Work out the finished part from the listing and answer in its coordinate system (mm). Face numbers are marked on the shaded views. A direction names the side the tool comes from. Give positions to 0.01 mm unless a question says otherwise; leave off trailing zeros. Loops run counter-clockwise (first coordinate to the right, second up) from the corner with the lowest first, then second, coordinate; pieces in that order, holes last. Notation, with made-up numbers: (65, -35.5) - (88, -35.5) arc R15 cw to (88, -13.5) - close; hole circle Ø6 at (47, -9.75). An arc over 180 degrees is marked (long way). One line per item, written item: value.
from build123d import *

# Parameters (mm, degrees)
SKETCH1_W               = 48
SKETCH1_H               = 40
BOSS_EXTRUDE1_DEPTH     = 6
CUT_EXTRUDE1_DEPTH      = 34.466401061
CUT_EXTRUDE1_DEPTH_BACK = 34.466401061
SKETCH3_R               = 1.5
BOSS_EXTRUDE2_DEPTH     = 1.5
FILLET1_R               = 3


with BuildPart() as part:
    # Sketch1 → Boss-Extrude1 (new, symmetric)
    with BuildSketch(Plane(origin=(0, 0, 0), x_dir=(1, 0, 0), z_dir=(0, 1, 0))):
        Rectangle(SKETCH1_W, SKETCH1_H)
    extrude(amount=BOSS_EXTRUDE1_DEPTH, both=True)

    # Sketch2 → Cut-Extrude1 (cut, two sides: drawn at the far end of the back side and taken through both)
    with BuildSketch(Plane(origin=(0, 6, 0), x_dir=(1, 0, 0), z_dir=(0, 1, 0)).offset(-CUT_EXTRUDE1_DEPTH_BACK)):
        with BuildLine():
            Line((-24, 13), (-20.5, 13))
            ThreePointArc((-20.5, 13), (-18.025126266, 14.025126266), (-17, 16.5))
            Line((-17, 16.5), (-17, 20))
            Line((-17, 20), (-24, 20))
            Line((-24, 20), (-24, 13))
        make_face()
        with BuildLine():
            Line((24, -13), (20.5, -13))
            ThreePointArc((20.5, -13), (18.025126266, -14.025126266), (17, -16.5))
            Line((17, -16.5), (17, -20))
            Line((17, -20), (24, -20))
            Line((24, -20), (24, -13))
        make_face()
    extrude(amount=CUT_EXTRUDE1_DEPTH + CUT_EXTRUDE1_DEPTH_BACK, mode=Mode.SUBTRACT)

    # Sketch3 → Boss-Extrude2 (add, symmetric)
    # profile 1 of 2: a face of its own
    with BuildSketch(Plane(origin=(0, 0, 0), x_dir=(1, 0, 0), z_dir=(0, 1, 0))):
        with BuildLine():
            Line((24, -13), (20.5, -13))
            ThreePointArc((20.5, -13), (18.025126266, -14.025126266), (17, -16.5))
            Line((17, -16.5), (17, -20))
            Line((17, -20), (24, -20))
            Line((24, -20), (24, -13))
        make_face()
        with Locations(Location((20.5, -16.5, 0), (0, 0, 270))):
            Circle(SKETCH3_R, mode=Mode.SUBTRACT)
    # profile 2 of 2: a face of its own
    with BuildSketch(Plane(origin=(0, 0, 0), x_dir=(1, 0, 0), z_dir=(0, 1, 0))):
        with BuildLine():
            Line((-24, 13), (-20.5, 13))
            ThreePointArc((-20.5, 13), (-18.025126266, 14.025126266), (-17, 16.5))
            Line((-17, 16.5), (-17, 20))
            Line((-17, 20), (-24, 20))
            Line((-24, 20), (-24, 13))
        make_face()
        with Locations(Location((-20.5, 16.5, 0), (0, 0, 270))):
            Circle(SKETCH3_R, mode=Mode.SUBTRACT)
    extrude(amount=BOSS_EXTRUDE2_DEPTH, both=True)

    # Fillet1
    fillet1_edges = [part.edges().sort_by_distance(p)[0] for p in [
        (24, 0, 20),
        (-24, 0, 20),
        (24, 0, -20),
        (-24, 0, -20),
    ]]
    fillet(fillet1_edges, radius=FILLET1_R)


solid = part.part
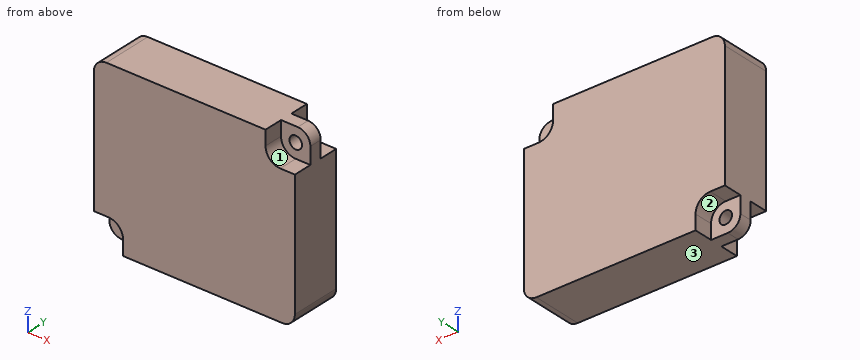
1. For the marked faces 1, 2 and 3, determine the directions among +Z, -Z, +X, -X, +Y, -Y from which every point of the face is accessible in a straight line to the end or side of a thin tool.
Output:
face 1: +Z, +X, -Y
face 2: -Z, -X, +Y
face 3: -Z, +X, -X, +Y, -Y
2. Flat-ended cylindrical pins translate along their axes: pin 1 Ø2.5 at (x, z) = (20.5, 16.5) entering from -Y; pin 2 Ø1 at (y, z) = (-3, -18.5) entering from -X; pin 3 Ø2 at (x, z) = (20.5, 18) entering from -Y; pin 4 Ø1 at (x, y) = (-22.5, -3) entering from -Z. Find the tip coordinate at first contact, or state that the pin passes through.
Output:
pin 1: passes through
pin 2: stops at x = -17
pin 3: stops at y = -1.5
pin 4: stops at z = -13
3. Section B-B (x = -18) is taken. Write down the section's boundary in (y, z), and give its area (3 significant figures).
Output:
outline: (-6, -14.05) - (-1.5, -14.05) - (-1.5, -20) - (1.5, -20) - (1.5, -14.05) - (6, -14.05) - (6, 20) - (-6, 20) - close
area: 426 mm²
4. Section A-A (y = 3) is taken. Write down the section's boundary in (x, z).
Output:
outline: (-24, -13) - (-20.5, -13) arc R3.5 cw to (-17, -16.5) - (-17, -20) - (21, -20) arc R3 ccw to (24, -17) - (24, 13) - (20.5, 13) arc R3.5 cw to (17, 16.5) - (17, 20) - (-21, 20) arc R3 ccw to (-24, 17) - close
5. Find the intervals of material crossed by line 1 along X through (y, z) = (0.05, -16.5); line 2 along X through (y, z) = (0.5, 16.5); line 3 along X through (y, z) = (-5, 16.5), in increasing order.
Output:
line 1: x = -24 to -22, -19 to 24
line 2: x = -24 to 19, 22 to 24
line 3: x = -24 to 17
